Autodesk Inventor part; units mm, degrees
ref_plane "Work Plane1" through (-7.1, 0, -96) normal (0, 0, -1) x (0, 1, 0)
ref_plane "Work Plane2" through (-7.1, -33.8, -97.5) normal (0, 0, -1) x (0, 1, 0)
ref_plane "Work Plane3" through (-7.1, -33.8, 1.5) normal (0, 0, 1) x (1, 0, 0)
sketch "Sketch1" plane through (0, 0, 0) normal (0, 0, 1) x (1, 0, 0)
  line L0 (0, 50.1071) -> (-7.1, 57.2071)
  line L1 (-7.1, 57.2071) -> (-7.1, 0)
  line L2 (0, 0) -> (-7.1, 0)
  line L3 (0, 50.1071) -> (0, 0)
  circle A0 centre (6, -18.6) radius 16.1
  line L4 (-10.1, -18.6) -> (-10.1, 64.4833)
  line L5 (-7.1, 57.2071) -> (-10.1, 60.2071)
  line L6 (-10.1, 60.2071) -> (2.6279, 47.4792)
  line L7 (2.6279, 47.4792) -> (4.7492, 49.6005)
  line L8 (4.7492, 49.6005) -> (-14.184, 68.5338)
  line L9 (-10.1, 64.4833) -> (-10.1, 67.3257)
  point P0 (-10.1, 64.4498)
  dimension "d0" = 18
  dimension "d1" = 3
ref_plane "Work Plane1" through (-7.1, 0, -96) normal (0, 0, -1) x (0, 1, 0)
extrude "Extrusion1" add sketch "Sketch1" against normal up to surface (96 mm away) contours L0 L5 L4 L8 L7 L6
sketch "Sketch2" plane through (-10.1, 64.4498, -96) normal (0.7071, 0.7071, 0) x (-0.7071, 0.7071, 0)
  circle A0 centre (-14.7131, 28.1488) radius 1.5
  circle A1 centre (-14.7131, 67.8512) radius 1.5
  point P0 (-52.7147, 96)
extrude "Extrusion2" cut sketch "Sketch2" against normal through all
sketch "Sketch3" plane through (-10.1, 60.2071, -96) normal (0, 0, -1) x (-1, 0, 0)
  line L0 (0, 4.2426) -> (0, 0)
  line L1 (-14.8492, -10.6066) -> (0, 4.2426)
  line L2 (-12.7279, -12.7279) -> (-14.8492, -10.6066)
  line L3 (0, 0) -> (-12.7279, -12.7279)
  point P0 (-10.1, -60.2071)
ref_plane "Work Plane2" through (-7.1, -33.8, -97.5) normal (0, 0, -1) x (0, 1, 0)
extrude "Extrusion3" add sketch "Sketch3" along normal up to surface (1.5 mm away)
sketch "Sketch4" plane through (0, 0, 0) normal (0, 0, 1) x (1, 0, 0)
  line L0 (4.7492, 49.6005) -> (-10.1, 64.4498)
  line L1 (-10.1, 64.4498) -> (-10.1, 60.2071)
  line L2 (-10.1, 60.2071) -> (2.6279, 47.4792)
  line L3 (2.6279, 47.4792) -> (4.7492, 49.6005)
  point P0 (0, 0)
ref_plane "Work Plane3" through (-7.1, -33.8, 1.5) normal (0, 0, 1) x (1, 0, 0)
extrude "Extrusion4" add sketch "Sketch4" along normal up to surface (1.5 mm away)
sketch "Sketch5" plane through (-10.1, 60.2071, 1.5) normal (0, 0, 1) x (1, 0, 0)
  line L0 (0, 4.2426) -> (14.8492, -10.6066)
  line L1 (0, 0) -> (0, 4.2426)
  line L2 (12.7279, -12.7279) -> (0, 0)
  line L3 (14.8492, -10.6066) -> (12.7279, -12.7279)
  point P0 (10.1, -60.2071)
ref_plane "Work Plane4" through (-8, -1.3502, 2.5) normal (0, 0, 1) x (1, 0, 0)
extrude "Extrusion5" add sketch "Sketch5" along normal up to surface (1 mm away)
properties part number "nozyk"
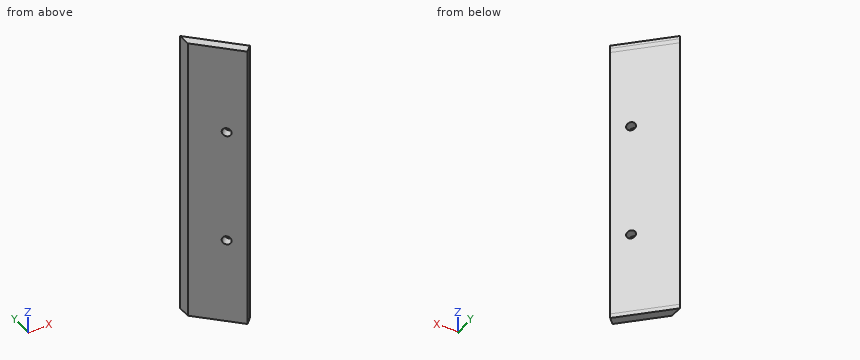
Input: part model. Units: mm. Frame: model coordinates. Round coordinates to 2 decimals unless told otherwise and drop trailing zeros. Write each loop counter-clockwise with the first axis right and the second up, starting at its lowest first coordinate (ties: lowest second). Pieces come first, ordered by that corner, then holes.
1) Cut plane B-B (z = -40.5). Return the cut outline in (x, y).
2) Ray query, L1, parallel to Y at x = -0.75, z = -74; L2, parallel to Z at x = -1.25, y = 51.75; L3, parallel to Y at x = 3, z = -20. Return the intervals inside material, ascending.
3) Contact query for flat-ended pins moving along their axis: P1, Ø1, axis at x = -7.5, z = -15.5, coming from the +Y side; P2, Ø7.5, axis at x = 0.5, y = 55.5, coming from the +Z side; P3, Ø3, axis at y = 49.5, z = -70.5, coming from the -X side; P4, Ø1, axis at x = -7.5, z = -82.5, coming from the -Y side. Output: stop coordinate, or through.
Geometry says:
1. outline: (-10.1, 60.21) - (2.63, 47.48) - (4.75, 49.6) - (-10.1, 64.45) - close
2. L1: y = 50.86 to 55.1
2. L2: z = -97.5 to -69.26, -66.45 to -29.55, -26.74 to 2.5
2. L3: y = 47.85 to 51.35
3. P1: stops at y = 62.35
3. P2: stops at z = 2.5
3. P3: stops at x = -0.89
3. P4: stops at y = 57.11
